from build123d import *

# Parameters (mm, degrees)
BOSS_EXTRUDE1_DEPTH   = 3
BOSS_EXTRUDE1_2_DEPTH = 3
SKETCH1_W             = 23.4
SKETCH1_H             = 29
SKETCH1_R             = 1
BOSS_EXTRUDE1_3_DEPTH = 3
FILLET1_R             = 2
SKETCH5_R             = 1.44
CUT_EXTRUDE3_DEPTH    = 10
CUT_EXTRUDE4_DEPTH    = 10
SKETCH8_R             = 1
CUT_EXTRUDE5_DEPTH    = 10
SKETCH9_R             = 3.026992654
BOSS_EXTRUDE3_DEPTH   = 3
SKETCH10_R            = 1.95
CUT_EXTRUDE6_DEPTH    = 10
SKETCH13_W            = 23.4
SKETCH13_H            = 29
SKETCH13_R            = 1.95
BOSS_EXTRUDE4_DEPTH   = 3


with BuildPart() as part:
    # Sketch1 → Boss-Extrude1 (new body)
    with BuildSketch(Plane(origin=(0, 0, 0), x_dir=(1, 0, 0), z_dir=(0, 1, 0))):
        with BuildLine():
            add(Edge.make_bspline(
                [(19.180993887, -14.242526212), (19.80083761, -12.341053413), (17.899318471, -11.721194585), (17.279474749, -13.622667384), (16.659631026, -15.524140184), (18.561150164, -16.143999012), (19.180993887, -14.242526212)],
                knots=[0, 0, 0, 0, 0.5, 0.5, 0.5, 1, 1, 1, 1], degree=3, weights=[1, 0.333333333, 0.333333333, 1, 0.333333333, 0.333333333, 1]))
        make_face()
    extrude(amount=BOSS_EXTRUDE1_DEPTH)


with BuildPart() as body_2:
    # Sketch1 → Boss-Extrude1 2 (new body)
    with BuildSketch(Plane(origin=(0, 0, 0), x_dir=(1, 0, 0), z_dir=(0, 1, 0))):
        with BuildLine():
            add(Edge.make_bspline(
                [(22.488505608, -4.096188772), (23.108349331, -2.194715972), (21.206830193, -1.574857144), (20.58698647, -3.476329943), (19.967142747, -5.377802743), (21.868661885, -5.997661571), (22.488505608, -4.096188772)],
                knots=[0, 0, 0, 0, 0.5, 0.5, 0.5, 1, 1, 1, 1], degree=3, weights=[1, 0.333333333, 0.333333333, 1, 0.333333333, 0.333333333, 1]))
        make_face()
    extrude(amount=BOSS_EXTRUDE1_2_DEPTH)


with BuildPart() as body_3:
    # Sketch1 → Boss-Extrude1 3 (new body)
    with BuildSketch(Plane(origin=(0, 0, 0), x_dir=(1, 0, 0), z_dir=(0, 1, 0))):
        Rectangle(SKETCH1_W, SKETCH1_H)
        with Locations(Location((9, 8.9, 0), (0, 0, 270))):
            Circle(SKETCH1_R, mode=Mode.SUBTRACT)
        with Locations(Location((9, -8.5, 0), (0, 0, 90))):
            Circle(SKETCH1_R, mode=Mode.SUBTRACT)
        with Locations(Location((-9, -8.5, 0), (0, 0, 90))):
            Circle(SKETCH1_R, mode=Mode.SUBTRACT)
        with Locations(Location((1.7, -8.5, 0), (0, 0, 90))):
            Circle(SKETCH1_R, mode=Mode.SUBTRACT)
    extrude(amount=BOSS_EXTRUDE1_3_DEPTH)

    # Fillet1
    fillet1_edges = [body_3.edges().sort_by_distance(p)[0] for p in [
        (11.7, 1.5, 14.5),
        (-11.7, 1.5, 14.5),
        (-11.7, 1.5, -14.5),
        (11.7, 1.5, -14.5),
    ]]
    fillet(fillet1_edges, radius=FILLET1_R)

    # Sketch5 → Cut-Extrude3 (cut)
    with BuildSketch(Plane.XZ):
        with Locations(Location((-2.145634177, 3.61037734, 0), (0, 0, 270))):
            Circle(SKETCH5_R)
    extrude(amount=-CUT_EXTRUDE3_DEPTH, mode=Mode.SUBTRACT)

    # Sketch8 → Cut-Extrude5 (cut)
    with BuildSketch(Plane(origin=(0, 3, 0), x_dir=(1, 0, 0), z_dir=(0, 1, 0))):
        with Locations(Location((1.7, 8.9, 0), (0, 0, 270))):
            Circle(SKETCH8_R)
        with Locations(Location((-9, 8.9, 0), (0, 0, 270))):
            Circle(SKETCH8_R)
    extrude(amount=-CUT_EXTRUDE5_DEPTH, mode=Mode.SUBTRACT)

    # Sketch9 → Boss-Extrude3 (add)
    with BuildSketch(Plane(origin=(0, 3, 0), x_dir=(1, 0, 0), z_dir=(0, 1, 0))):
        with Locations((-2.145634177, -3.61037734)):
            Circle(SKETCH9_R)
    extrude(amount=-BOSS_EXTRUDE3_DEPTH)

    # Sketch10 → Cut-Extrude6 (cut)
    with BuildSketch(Plane(origin=(0, 3, 0), x_dir=(1, 0, 0), z_dir=(0, 1, 0))):
        with Locations(Location((-2.328177417, -0.1, 0), (0, 0, 270))):
            Circle(SKETCH10_R)
    extrude(amount=-CUT_EXTRUDE6_DEPTH, mode=Mode.SUBTRACT)

    # Sketch13 → Boss-Extrude4 (add)
    with BuildSketch(Plane(origin=(0, 3, 0), x_dir=(1, 0, 0), z_dir=(0, 1, 0))):
        Rectangle(SKETCH13_W, SKETCH13_H)
        with Locations(Location((-2.328177417, -0.1, 0), (0, 0, 270))):
            Circle(SKETCH13_R, mode=Mode.SUBTRACT)
    extrude(amount=-BOSS_EXTRUDE4_DEPTH)


with BuildPart() as cut_extrude4_tool:
    # Sketch7 → Cut-Extrude4 (new body)
    with BuildSketch(Plane(origin=(0, 3, 0), x_dir=(1, 0, 0), z_dir=(0, 1, 0))):
        with BuildLine():
            add(Edge.make_bspline(
                [(19.180993887, -14.242526212), (19.80083761, -12.341053413), (17.899318471, -11.721194585), (17.279474749, -13.622667384), (16.659631026, -15.524140184), (18.561150164, -16.143999012), (19.180993887, -14.242526212)],
                knots=[0, 0, 0, 0, 0.5, 0.5, 0.5, 1, 1, 1, 1], degree=3, weights=[1, 0.333333333, 0.333333333, 1, 0.333333333, 0.333333333, 1]))
        make_face()
        with BuildLine():
            add(Edge.make_bspline(
                [(22.488505608, -4.096188772), (23.108349331, -2.194715972), (21.206830193, -1.574857144), (20.58698647, -3.476329943), (19.967142747, -5.377802743), (21.868661885, -5.997661571), (22.488505608, -4.096188772)],
                knots=[0, 0, 0, 0, 0.5, 0.5, 0.5, 1, 1, 1, 1], degree=3, weights=[1, 0.333333333, 0.333333333, 1, 0.333333333, 0.333333333, 1]))
        make_face()
    extrude(amount=-CUT_EXTRUDE4_DEPTH)


with BuildPart() as part_1:
    add(part.part)

    # Cut-Extrude4: cut by cut_extrude4_tool
    add(cut_extrude4_tool.part, mode=Mode.SUBTRACT)


with BuildPart() as body_2_1:
    add(body_2.part)

    # Cut-Extrude4: cut by cut_extrude4_tool
    add(cut_extrude4_tool.part, mode=Mode.SUBTRACT)


solid = body_3.part
Part model, mm, in its own coordinate system. Coordinates: 2 decimals unless noted, no trailing zeros. Order: outer loops, then holes, each group sorted by start corner. A loop starts at its lowest first (then second) coordinate and runs counter-clockwise, first axis right, second up. Notation, with made-up numbers: M 17.5,48 L 60.5,48 A21 ccw 60.5,75 Z; hole C 55,76.5 d1. An arc over 180 degrees is marked long. One line per question, with ' | ' between items.
Q1. Two-plate mould, pull along X, no slides. Class faces 1 (the face through (0, 0, 0)), 2 (the face through (11.7, 1, 0)), 3 (the face through (-0.4, 1.5, -0.2)): +X half, -X half, draft (parallel to the pull), parting line (faces both ways), or undercut.
A:
face 1: draft | face 2: +X half | face 3: undercut
Q2. Drill centre lines: line 1 (X direction, y = 1.85, z = 0.1); line 2 (Z direction, x = -2, y = 0.6); line 3 (X direction, y = 0.25, z = 1.5). Where is each one in solid material? Low to high.
A:
line 1: x = -11.7 to -4.28, -0.38 to 11.7 | line 2: z = -14.5 to -1.82, 2.02 to 14.5 | line 3: x = -11.7 to -3.69, -0.97 to 11.7
Q3. Slice it at A-A (z = 0.1). Give the cut face in (x, y).
A:
outline: M -11.7,0 L -4.28,0 L -4.28,3 L -11.7,3 Z; M -0.38,0 L 11.7,0 L 11.7,3 L -0.38,3 Z
Q4. Slice it at B-B (y = 0.55). Give the cut face in (x, z).
A:
outline: M -11.7,-14.5 L 11.7,-14.5 L 11.7,14.5 L -11.7,14.5 Z; hole C -2.33,0.1 d3.9
